from build123d import *

# Parameters (mm, degrees)
F0_R     = 20
F1_DEPTH = 5
F2_R     = 15
F3_DEPTH = 0.1
F4_R     = 0.5
F5_R     = 1
F6_DEPTH = 0.5
F7_R     = 0.1


with BuildPart() as f1:
    # F0 (on Top) → F1 (new body)
    with BuildSketch(Plane.XY):
        Circle(F0_R)
    extrude(amount=F1_DEPTH)

    # F2 (on face) → F3 (join)
    with BuildSketch(Plane.XY.offset(5)):
        Circle(F2_R)
    extrude(amount=F3_DEPTH)

    # F4
    f4_edges = [f1.edges().sort_by_distance(p)[0] for p in [
        (-20, 0, 5),
    ]]
    fillet(f4_edges, radius=F4_R)

    # F5 (on face) → F6 (join)
    with BuildSketch(Plane.XY.offset(5.1)):
        Circle(F5_R)
    extrude(amount=F6_DEPTH)

    # F7
    f7_edges = [f1.edges().sort_by_distance(p)[0] for p in [
        (-1, 0, 5.6),
    ]]
    fillet(f7_edges, radius=F7_R)


solid = f1.part
Geometry check sheet. Reference: the model listing, model coordinates, mm. A direction names the side the tool comes from. Give positions to 0.01 mm unless a question says otherwise; leave off trailing zeros. Write each loop counter-clockwise with the first axis right and the second up, starting at its lowest first coordinate (ties: lowest second). Pieces come first, ordered by that corner, then holes. Notation, with made-up numbers: M -8.5,79.25 L 21.5,79.25 A24 cw 21.5,99.25 Z; hole C -16.5,-36.5 d3. An arc over 180 degrees is marked long. Answer as CSV lines item,"result". Start each with the question number.
Q1. Tool access check on faces 1 (the face through (10, -11.5, 5)), 2 (the face through (0, 0, 0)). Record the directions out of +Z, -Z, +X, -X, +Y, -Y that give a thin tool (end or side, any length) a straight path to the whole face; none if there is none.
Q2. Section check A-A, the plane x = 0. Record the cut outline in (y, z), then the cut area to 3 significant figures.
Q3. Material ranges on L1, parallel to Z at x = -5, y = 16.5; L2, parallel to Z at x = -3.5, y = 9.5; L3, parallel to Y at x = -0.5, z = 1.95, recorded low to high.
Q4. Section check C-C, the plane z = 3.5. Record the cut outline in (x, y).
Q5. Go/stop test with flat-tipped pins: pin 1 (3 mm diameter, centred on x = -8.5, z = 4, fed in from -Y) (3 decimals); pin 2 (8 mm diameter, centred on x = 6, y = 5.5, fed in from +Z); pin 3 (1 mm diameter, centred on x = 7, z = 4.5, fed in from +Y). Record where each tip stops, or that it passes through.
Geometry says:
1,face 1,"+Z"
1,face 2,"-Z, +X, -X, +Y, -Y"
2,outline,"M -20,0 L 20,0 L 20,4.5 A0.5 ccw 19.5,5 L 15,5 L 15,5.1 L 1,5.1 L 1,5.5 A0.1 ccw 0.9,5.6 L -0.9,5.6 A0.1 ccw -1,5.5 L -1,5.1 L -15,5.1 L -15,5 L -19.5,5 A0.5 ccw -20,4.5 Z"
2,area,"204 mm^2"
3,L1,"0 to 5"
3,L2,"0 to 5.1"
3,L3,"-19.99 to 19.99"
4,outline,"C 0,0 d40"
5,pin 1,"y = -18.735"
5,pin 2,"z = 5.1"
5,pin 3,"y = 18.91"
